from build123d import *

# Parameters (mm, degrees)
BOX_W                  = 22
BOX_H                  = 1
BOX_DEPTH              = 0.8
BOX001_W               = 22
BOX001_H               = 1
BOX001_DEPTH           = 0.8
BOX001_PLACEMENT_ANGLE = 60
BOX002_W               = 22
BOX002_H               = 1
BOX002_DEPTH           = 0.8
BOX002_PLACEMENT_ANGLE = -60
CYLINDER003_R          = 14
CYLINDER003_DEPTH      = 4
CYLINDER002_R          = 16
CYLINDER002_DEPTH      = 4
CYLINDER001_R          = 10
CYLINDER001_DEPTH      = 1
CYLINDER_R             = 20
CYLINDER_DEPTH         = 0.8


with BuildPart() as box:
    # Box → Box (new body)
    with BuildSketch(Plane(origin=(-11, 0, 0), x_dir=(1, 0, 0), z_dir=(0, 0, 1))):
        with Locations((11, 0.5)):
            Rectangle(BOX_W, BOX_H)
    extrude(amount=BOX_DEPTH)


with BuildPart() as box001:
    # Box001 → Box001 (new body)
    with BuildSketch(Plane.XY):
        with Locations((11, 0.5)):
            Rectangle(BOX001_W, BOX001_H)
    extrude(amount=BOX001_DEPTH)


with BuildPart() as box001_1:
    # Box001 placement: moved
    add(box001.part.moved(Location((-6, -10, 0))).rotate(Axis((-6, -10, 0), (0, 0, 1)), BOX001_PLACEMENT_ANGLE))


with BuildPart() as box002:
    # Box002 → Box002 (new body)
    with BuildSketch(Plane.XY):
        with Locations((11, 0.5)):
            Rectangle(BOX002_W, BOX002_H)
    extrude(amount=BOX002_DEPTH)


with BuildPart() as box002_1:
    # Box002 placement: moved
    add(box002.part.moved(Location((-6, 9, 0))).rotate(Axis((-6, 9, 0), (0, 0, 1)), BOX002_PLACEMENT_ANGLE))


with BuildPart() as shoulder_in:
    # Cylinder003 → Cylinder003 (new body)
    with BuildSketch(Plane.XY):
        Circle(CYLINDER003_R)
    extrude(amount=CYLINDER003_DEPTH)


with BuildPart() as shoulder:
    # Cylinder002 → Cylinder002 (new body)
    with BuildSketch(Plane.XY):
        Circle(CYLINDER002_R)
    extrude(amount=CYLINDER002_DEPTH)

    # Cut001: cut shoulder_in
    add(shoulder_in.part, mode=Mode.SUBTRACT)


with BuildPart() as hole:
    # Cylinder001 → Cylinder001 (new body)
    with BuildSketch(Plane.XY):
        Circle(CYLINDER001_R)
    extrude(amount=CYLINDER001_DEPTH)


with BuildPart() as bottom:
    # Cylinder → Cylinder (new body)
    with BuildSketch(Plane.XY):
        Circle(CYLINDER_R)
    extrude(amount=CYLINDER_DEPTH)

    # Cut: cut hole
    add(hole.part, mode=Mode.SUBTRACT)

    # Fusion: union Box, Box001, Box002, shoulder
    add(box.part)
    add(box001_1.part)
    add(box002_1.part)
    add(shoulder.part)


solid = bottom.part
Input: part model. Units: mm. Frame: model coordinates. A direction names the side the tool comes from. Coordinates: 2 decimals unless noted, no trailing zeros. Loops run counter-clockwise (first coordinate to the right, second up) from the corner with the lowest first, then second, coordinate; pieces in that order, holes last.
(1) Set-up query: faces 4 (the face through (0, 0, 0)), 5 (the face through (0, 0, 0.8)), 6 (the face through (-2.875, -4.587, 0.394)). Return all of +Z, -Z, +X, -X, +Y, -Y with unobstructed straight access to the full face (end or side cutting, diameter ignored); none if empty.
(2) First-contact query: pin 1 Ø2 at (y, z) = (10, 1.5) entering from +X; pin 2 Ø12 at (x, y) = (1.5, -3.5) entering from +Z; pin 3 Ø0.9 at (x, z) = (4, 0.5) entering from -Y; pin 4 Ø6 at (x, y) = (11, -12.5) entering from -Z. Flat tips, straight axial feed; report the tip coordinate or a pass-through.
(3) Section A-A on y = 2. Return the cut outline in (x, z).
(4) Section C-C on z = 2.4. Return the cut outline in (x, y).
(5) Pull-direction query (X, two-part tool) for faces 1 (the face through (-3.47, -15.62, 2.38)), 2 (the face through (7.14, 14.49, 0.8)), 3 (the face through (-3.723, -4.056, 0.394)); classes: released by +X, released by -X, zero draft, split by the parting line, or undercut.
(6) Section D-D on x = 1.5. Return the cut outline in (y, z), then the cut area to 3 significant figures.
(7) Material intervals for probe 1 along X at (y, z) = (0, 2.9); probe 2 along X at (y, z) = (2, 0.75), sorted ascending.
(8) Section B-B on x = -3. Return the cut outline in (y, z), then the cut area to 3 significant figures.
Data:
1. face 4: -Z, +X, -X, +Y, -Y
1. face 5: +Z
1. face 6: +Z, -Z
2. pin 1: stops at x = 17.71
2. pin 2: stops at z = 0.8
2. pin 3: stops at y = -19.68
2. pin 4: stops at z = 0
3. outline: (-19.9, 0) - (-9.8, 0) - (-9.8, 0.8) - (-13.86, 0.8) - (-13.86, 4) - (-15.87, 4) - (-15.87, 0.8) - (-19.9, 0.8) - close; (-1.96, 0) - (-0.8, 0) - (-0.8, 0.8) - (-1.96, 0.8) - close; (-0.23, 0) - (0.93, 0) - (0.93, 0.8) - (-0.23, 0.8) - close; (9.8, 0) - (19.9, 0) - (19.9, 0.8) - (15.87, 0.8) - (15.87, 4) - (13.86, 4) - (13.86, 0.8) - (9.8, 0.8) - close
4. outline: circle Ø32 at (0, 0); hole circle Ø28 at (0, 0)
5. face 1: split by the parting line
5. face 2: zero draft
5. face 3: undercut
6. outline: (-19.94, 0) - (-9.89, 0) - (-9.89, 0.8) - (-13.92, 0.8) - (-13.92, 4) - (-15.93, 4) - (-15.93, 0.8) - (-19.94, 0.8) - close; (-3.99, 0) - (-1.99, 0) - (-1.99, 0.8) - (-3.99, 0.8) - close; (0, 0) - (1, 0) - (1, 0.8) - (0, 0.8) - close; (2.99, 0) - (4.99, 0) - (4.99, 0.8) - (2.99, 0.8) - close; (9.89, 0) - (19.94, 0) - (19.94, 0.8) - (15.93, 0.8) - (15.93, 4) - (13.92, 4) - (13.92, 0.8) - (9.89, 0.8) - close
6. area: 33.0 mm2
7. probe 1: x = -16 to -14, 14 to 16
7. probe 2: x = -19.9 to -9.8, -1.96 to -0.8, -0.23 to 0.93, 9.8 to 19.9
8. outline: (-19.77, 0) - (-9.54, 0) - (-9.54, 0.8) - (-13.67, 0.8) - (-13.67, 4) - (-15.72, 4) - (-15.72, 0.8) - (-19.77, 0.8) - close; (-4.8, 0) - (-2.8, 0) - (-2.8, 0.8) - (-4.8, 0.8) - close; (0, 0) - (1, 0) - (1, 0.8) - (0, 0.8) - close; (3.8, 0) - (5.8, 0) - (5.8, 0.8) - (3.8, 0.8) - close; (9.54, 0) - (19.77, 0) - (19.77, 0.8) - (15.72, 0.8) - (15.72, 4) - (13.67, 4) - (13.67, 0.8) - (9.54, 0.8) - close
8. area: 33.4 mm2
